Read the model definition and answer for the solid it produces. Units are mm, in the model's axes. A direction names the side the tool comes from. Coordinates: 2 decimals unless noted, no trailing zeros. Loops run counter-clockwise (first coordinate to the right, second up) from the corner with the lowest first, then second, coordinate; pieces in that order, holes last.
from build123d import *

# Parameters (mm, degrees)
BOX031_W     = 53
BOX031_H     = 7
BOX031_DEPTH = 55
BOX029_W     = 47
BOX029_H     = 12
BOX029_DEPTH = 50
BOX030_W     = 53
BOX030_H     = 11
BOX030_DEPTH = 55


with BuildPart() as cube030:
    # Box031 → Box031 (new body)
    with BuildSketch(Plane(origin=(-12, 3, -2.5), x_dir=(1, 0, 0), z_dir=(0, 0, 1))):
        with Locations((26.5, 3.5)):
            Rectangle(BOX031_W, BOX031_H)
    extrude(amount=BOX031_DEPTH)


with BuildPart() as cube028:
    # Box029 → Box029 (new body)
    with BuildSketch(Plane(origin=(-9, -8, 0), x_dir=(1, 0, 0), z_dir=(0, 0, 1))):
        with Locations((23.5, 6)):
            Rectangle(BOX029_W, BOX029_H)
    extrude(amount=BOX029_DEPTH)


with BuildPart() as fusion096:
    # Box030 → Box030 (new body)
    with BuildSketch(Plane(origin=(-12, -8, -2.5), x_dir=(1, 0, 0), z_dir=(0, 0, 1))):
        with Locations((26.5, 5.5)):
            Rectangle(BOX030_W, BOX030_H)
    extrude(amount=BOX030_DEPTH)

    # Cut045020: cut Cube028
    add(cube028.part, mode=Mode.SUBTRACT)

    # Fusion096: union Cube030
    add(cube030.part)


solid = fusion096.part
Q1. Determine the mould class of faces 1 (the face through (-12, 1, 25)), 2 (the face through (14, 10, 25)), 3 (the face through (-9, -3, 25)) for opening direction X: +X half, -X half, draft (parallel to the pull), parting line (faces both ways), or undercut.
Findings below:
face 1: -X half
face 2: draft
face 3: undercut
Q2. A flat-ended cylindrical pin translates along its axis: pin 1 Ø8 at (x, z) = (0.5, 25) entering from -Y. Find the tip coordinate at first contact, or state that the pin passes through.
Findings below:
pin 1: stops at y = 3
Q3. A cutting plane is placed at A-A (z = 18). Give the vertices of the cut face in (x, y), then the cut area to 3 significant figures.
Findings below:
outline: (-12, -8) - (-9, -8) - (-9, 3) - (38, 3) - (38, -8) - (41, -8) - (41, 10) - (-12, 10) - close
area: 437 mm2
Q4. A cutting plane is placed at B-B (y = 1). Give the vertices of the cut face in (x, z).
Findings below:
outline: (-12, -2.5) - (41, -2.5) - (41, 52.5) - (-12, 52.5) - close; hole (-9, 0) - (38, 0) - (38, 50) - (-9, 50) - close
Q5. A cutting plane is placed at C-C (x = 12.5). Give the vertices of the cut face in (y, z), then the cut area to 3 significant figures.
Findings below:
outline: (-8, -2.5) - (10, -2.5) - (10, 52.5) - (-8, 52.5) - (-8, 50) - (3, 50) - (3, 0) - (-8, 0) - close
area: 440 mm2
Q6. Which of the six approach directions +Z, -Z, +X, -X, +Y, -Y give full straight-line access (tool end or side, diameter ignored) to faces 4 (the face through (14, -2, 50)), 5 (the face through (14, 1, -2.5))?
Findings below:
face 4: -Y
face 5: -Z, +X, -X, +Y, -Y
Q7. Straight lines are drawn through the part: probe 1 along X at (y, z) = (1.75, 32); probe 2 along Z at (x, y) = (20, -0.75); probe 3 along Y at (x, z) = (8.5, 42). For each, find the intervals that lie inside material, in ascending order.
Findings below:
probe 1: x = -12 to -9, 38 to 41
probe 2: z = -2.5 to 0, 50 to 52.5
probe 3: y = 3 to 10
